```python
from build123d import *

# Parameters (mm, degrees)
F3_DEPTH = 3


with BuildPart() as f1:
    # F0 (on Right) → F1 (revolve)
    with BuildSketch(Plane.YZ):
        Polygon((0, 6.5), (7, 6.5), (7, 8.05), (12.5, 8.05), (12.5, 19), (10, 18.5), (7.5, 18.5), (5, 18), (2.5, 18), (0, 17.5), (0, 14.5), (-3, 14.5), (-3, 10.05), (0, 10.05), align=None)
    revolve(axis=Axis((0, 20.883844794, 0), (0, 1, 0)))

    # F2 (on face) → F3 (cut)
    with BuildSketch(Plane.XZ.offset(3)):
        with BuildLine():
            ThreePointArc((1, 14.4654761415), (0, 14.5), (-1, 14.4654761415))
            ThreePointArc((-1, 14.4654761415), (0, 13.4994042291), (1, 14.4654761415))
        make_face()
        with BuildLine():
            ThreePointArc((-4.9700937486, 13.6216066648), (-5.8976813246, 13.2464091358), (-6.7971846639, 12.8081333786))
            ThreePointArc((-6.7971846639, 12.8081333786), (-5.4907023597, 12.3323194143), (-4.9700937486, 13.6216066648))
        make_face()
        with BuildLine():
            ThreePointArc((-10.0808131363, 10.4224376473), (-10.7755999694, 9.7023937922), (-11.419074349, 8.9361479963))
            ThreePointArc((-11.419074349, 8.9361479963), (-10.0320123999, 9.0328645373), (-10.0808131363, 10.4224376473))
        make_face()
        with BuildLine():
            ThreePointArc((-13.4484683513, 5.4211344757), (-13.7903194863, 4.4807464184), (-14.0665023401, 3.5190214432))
            ThreePointArc((-14.0665023401, 3.5190214432), (-12.8386963582, 4.1715453207), (-13.4484683513, 5.4211344757))
        make_face()
        with BuildLine():
            ThreePointArc((-14.4907612129, -0.5175320961), (-14.4205674828, -1.5156627174), (-14.2817042864, -2.5065758869))
            ThreePointArc((-14.2817042864, -2.5065758869), (-13.4254530802, -1.4110719791), (-14.4907612129, -0.5175320961))
        make_face()
        with BuildLine():
            ThreePointArc((-13.0274698164, -6.366712667), (-12.5573683549, -7.25), (-12.0274698164, -8.0987634745))
            ThreePointArc((-12.0274698164, -8.0987634745), (-11.6908269983, -6.7497021145), (-13.0274698164, -6.366712667))
        make_face()
        with BuildLine():
            ThreePointArc((-9.3116105377, -11.1150307779), (-8.5228861582, -11.7307464184), (-7.693576549, -12.2906012825))
            ThreePointArc((-7.693576549, -12.2906012825), (-7.9347507206, -10.9212474353), (-9.3116105377, -11.1150307779))
        make_face()
        with BuildLine():
            ThreePointArc((-3.9856892038, -13.9414590905), (-3.0147195169, -14.1831402106), (-2.0293940023, -14.3572824721))
            ThreePointArc((-2.0293940023, -14.3572824721), (-2.8066839583, -13.204409858), (-3.9856892038, -13.9414590905))
        make_face()
        with BuildLine():
            ThreePointArc((2.0293940023, -14.3572824721), (3.0147195169, -14.1831402106), (3.9856892038, -13.9414590905))
            ThreePointArc((3.9856892038, -13.9414590905), (2.8066839583, -13.204409858), (2.0293940023, -14.3572824721))
        make_face()
        with BuildLine():
            ThreePointArc((7.693576549, -12.2906012825), (8.5228861582, -11.7307464184), (9.3116105377, -11.1150307779))
            ThreePointArc((9.3116105377, -11.1150307779), (7.9347507206, -10.9212474353), (7.693576549, -12.2906012825))
        make_face()
        with BuildLine():
            ThreePointArc((12.0274698164, -8.0987634745), (12.5573683549, -7.25), (13.0274698164, -6.366712667))
            ThreePointArc((13.0274698164, -6.366712667), (11.6908269983, -6.7497021145), (12.0274698164, -8.0987634745))
        make_face()
        with BuildLine():
            ThreePointArc((14.2817042864, -2.5065758869), (14.4205674828, -1.5156627174), (14.4907612129, -0.5175320961))
            ThreePointArc((14.4907612129, -0.5175320961), (13.4254530802, -1.4110719791), (14.2817042864, -2.5065758869))
        make_face()
        with BuildLine():
            ThreePointArc((14.0665023401, 3.5190214432), (13.7903194863, 4.4807464184), (13.4484683513, 5.4211344757))
            ThreePointArc((13.4484683513, 5.4211344757), (12.8386963582, 4.1715453207), (14.0665023401, 3.5190214432))
        make_face()
        with BuildLine():
            ThreePointArc((11.419074349, 8.9361479963), (10.7755999694, 9.7023937922), (10.0808131363, 10.4224376473))
            ThreePointArc((10.0808131363, 10.4224376473), (10.0320123999, 9.0328645373), (11.419074349, 8.9361479963))
        make_face()
        with BuildLine():
            ThreePointArc((6.7971846639, 12.8081333786), (5.8976813246, 13.2464091358), (4.9700937486, 13.6216066648))
            ThreePointArc((4.9700937486, 13.6216066648), (5.4907023597, 12.3323194143), (6.7971846639, 12.8081333786))
        make_face()
    extrude(amount=-F3_DEPTH, mode=Mode.SUBTRACT)


solid = f1.part
```
Could you check a few things on this model? Use its own coordinates, in mm. A direction names the side the tool comes from. Round coordinates to 2 decimals unless told otherwise and drop trailing zeros. Loops run counter-clockwise (first coordinate to the right, second up) from the corner with the lowest first, then second, coordinate; pieces in that order, holes last. Notation, with made-up numbers: M 78,-11.5 L 115,-11.5 A17 ccw 115,15.5 Z; hole C 39,57.25 d7. An arc over 180 degrees is marked long. Put each result on its own line as item: value.
Q1. Imagine slicing it at B-B (z = 0). Write out the boundary of the cut face in (x, y).
Check result:
outline: M -19,12.5 L -18.5,10 L -18.5,7.5 L -18,5 L -18,2.5 L -17.5,0 L -14.5,0 L -14.5,-3 L -10.05,-3 L -10.05,0 L -6.5,0 L -6.5,7 L -8.05,7 L -8.05,12.5 Z; M 6.5,0 L 10.05,0 L 10.05,-3 L 14.5,-3 L 14.5,0 L 17.5,0 L 18,2.5 L 18,5 L 18.5,7.5 L 18.5,10 L 19,12.5 L 8.05,12.5 L 8.05,7 L 6.5,7 Z
Q2. I need wall thicknesses on probe 1 along X at (y, z) = (-1.05, 0); probe 2 along X at (y, z) = (3, 0); probe 3 along Y at (x, z) = (-13.5, -6.5). Which ranges of each line are inside material? Lowest first, please.
Check result:
probe 1: -14.5 to -10.05, 10.05 to 14.5
probe 2: -18 to -6.5, 6.5 to 18
probe 3: 0 to 12.5
Q3. Thinking about a two-plate mould opening in Z: for faces 1 (the face through (-8.2, 12.5, 0.3)), 2 (the face through (17.847, 3.732, -2.343)), 3 (the face through (5.47, -1.52, 12.34)), which applies, released by +Z, released by -Z, zero draft, split by the parting line, or undercut?
Check result:
face 1: zero draft
face 2: split by the parting line
face 3: undercut
Q4. Imagine slicing it at D-D (y = 9.5). Write out the boundary of the cut face in (x, z), then the cut area to 3 significant figures.
Check result:
outline: C 0,0 d37; hole C 0,0 d16.1
area: 872 mm2
Q5. On a 3-axis mill with a long thin cutter (end or side, diameter ignored), from which of +Z, -Z, +X, -X, +Y, -Y can I reach the whole of each face in a straight line? I mean faces 4 (the face through (5.924, -1.521, -13.235)), 5 (the face through (0, -1.5, -14.5)), 6 (the face through (2.418, 9.788, 7.678)), 7 (the face through (-3.043, -1.521, 14.177)), 8 (the face through (-7.92, -1.52, -10.93)). Say none if no direction works.
Check result:
face 4: -Z, +X, -Y
face 5: -Z, -Y
face 6: +Y
face 7: +Z, -X, -Y
face 8: -Y
Q6. For pin 1 (6 mm diameter, centred on x = -0.5, z = -0.5, fed in from -Y); pin 2 (4 mm diameter, centred on x = -7, y = 7.5, fed in from +Z); pin 3 (1.5 mm diameter, centred on x = 3, y = 6.5, fed in from +Z); pin 4 (5 mm diameter, centred on x = 8.5, y = 10, fed in from -Z), each with a flat end and sliding along its axis, tell me the tip position at first contact or that it passes through.
Check result:
pin 1: through
pin 2: z = 17.81
pin 3: z = 18.24
pin 4: z = -17.65
Q7. Imagine slicing it at A-A (x = 0). Write out the boundary of the cut face in (y, z), then the cut area to 3 significant figures.
Check result:
outline: M -3,-14.5 L 0,-14.5 L 0,-17.5 L 2.5,-18 L 5,-18 L 7.5,-18.5 L 10,-18.5 L 12.5,-19 L 12.5,-8.05 L 7,-8.05 L 7,-6.5 L 0,-6.5 L 0,-10.05 L -3,-10.05 Z; M -3,10.05 L 0,10.05 L 0,6.5 L 7,6.5 L 7,8.05 L 12.5,8.05 L 12.5,19 L 10,18.5 L 7.5,18.5 L 5,18 L 2.5,18 L 0,17.5 L 0,13.5 L -3,13.5 Z
area: 300 mm2
